Input: part model. Units: mm. Frame: model coordinates. Coordinates: 2 decimals unless noted, no trailing zeros. Loops run counter-clockwise (first coordinate to the right, second up) from the corner with the lowest first, then second, coordinate; pieces in that order, holes last.
(1) Section A-A, the plane y = 0. Return loops of the section in (x, z), then the cut area to 3 significant figures.
(2) Section C-C, the plane x = 162.5. Return loops of the section in (y, z), then the cut area to 3 significant figures.
(3) Contact query for flat-ended pins moving along their axis: P1, Ø2, axis at y = 5, z = -4, coming from the -X side; P2, Ø1.5, axis at x = 68, z = 4.5, coming from the -Y side; P3, Ø2, axis at x = 143, y = 6.5, coming from the -Z side; P4, Ø4, axis at x = 86, y = 3, coming from the -Z side. Output: stop coordinate, or through.
(4) Line query: L1, parallel to Z at x = 170.5, y = 0; L2, parallel to Z at x = 136.5, y = -4.5; L3, parallel to Y at x = 136.5, z = -6.5. Output: solid intervals per line, ascending.
Autodesk Inventor part; units mm, degrees
ref_plane "tube_front_XY" through (0, 0, 0) normal (1, 0, 0) x (0, 0, -1)
ref_plane "tube_front_YZ" through (0, 0, 0) normal (0, 0, -1) x (0, 1, 0)
ref_plane "tube_front_ZX" through (0, 0, 0) normal (0, 1, 0) x (1, 0, 0)
sketch "Sketch_1" plane through (0, 0, 0) normal (0, 0, 1) x (1, 0, 0)
  line L0 (260.4897, 0) -> (0, 0)
  arc A0 (-0.6395, 9.3472) -> (-0.6395, 9.1676) centre (-0.5497, 9.2574) ccw
  line L1 (-0.6395, 9.1676) -> (-0.381, 8.9091)
  line L2 (-0.381, 8.9091) -> (0, 8.9091)
  line L3 (0, 8.9091) -> (0.762, 9.671)
  line L4 (0.762, 9.671) -> (259.7277, 9.671)
  line L5 (259.7277, 9.671) -> (260.4897, 8.9091)
  line L6 (260.4897, 8.9091) -> (260.8707, 8.9091)
  line L7 (260.8707, 8.9091) -> (261.1292, 9.1676)
  arc A1 (261.1292, 9.1676) -> (261.1292, 9.3472) centre (261.0394, 9.2574) ccw
  line L8 (261.1292, 9.3472) -> (260.4443, 10.0321)
  arc A2 (260.4443, 10.0321) -> (259.9055, 10.2553) centre (259.9055, 9.4933) ccw
  line L9 (259.9055, 10.2553) -> (0.5842, 10.2553)
  arc A3 (0.5842, 10.2553) -> (0.0454, 10.0321) centre (0.5842, 9.4933) ccw
  line L10 (0.0454, 10.0321) -> (-0.6395, 9.3472)
revolve "Revolution1" add sketch "Sketch_1" angle 360 about axis through (260.4897, 0, 0) along (1, 0, 0)
ref_plane "tube_front_XY" through (0, 0, 0) normal (1, 0, 0) x (0, 0, -1)
ref_plane "tube_front_YZ" through (0, 0, 0) normal (0, 0, -1) x (0, 1, 0)
ref_plane "tube_front_ZX" through (0, 0, 0) normal (0, 1, 0) x (1, 0, 0)
ref_plane "tube_rear_XY" through (260.4897, 0, 0) normal (1, 0, 0) x (0, 0, -1)
ref_plane "tube_rear_YZ" through (260.4897, 0, 0) normal (0, 0, -1) x (0, 1, 0)
ref_plane "tube_rear_ZX" through (260.4897, 0, 0) normal (0, 1, 0) x (1, 0, 0)
ref_plane "cp1_XY" through (130.2449, 10.2553, 0) normal (1, 0, 0) x (0, 0, -1)
ref_plane "cp1_YZ" through (130.2449, 10.2553, 0) normal (0, 0, -1) x (0, 1, 0)
ref_plane "cp1_ZX" through (130.2449, 10.2553, 0) normal (0, 1, 0) x (1, 0, 0)
ref_plane "cp2_XY" through (130.2449, 0, -10.2553) normal (1, 0, 0) x (0, 0, -1)
ref_plane "cp2_YZ" through (130.2449, 0, -10.2553) normal (0, 0, -1) x (0, 1, 0)
ref_plane "cp2_ZX" through (130.2449, 0, -10.2553) normal (0, 1, 0) x (1, 0, 0)
ref_plane "cp3_XY" through (130.2449, -10.2553, 0) normal (1, 0, 0) x (0, 0, -1)
ref_plane "cp3_YZ" through (130.2449, -10.2553, 0) normal (0, 0, -1) x (0, 1, 0)
ref_plane "cp3_ZX" through (130.2449, -10.2553, 0) normal (0, 1, 0) x (1, 0, 0)
ref_plane "cp4_XY" through (130.2449, 0, 10.2553) normal (1, 0, 0) x (0, 0, -1)
ref_plane "cp4_YZ" through (130.2449, 0, 10.2553) normal (0, 0, -1) x (0, 1, 0)
ref_plane "cp4_ZX" through (130.2449, 0, 10.2553) normal (0, 1, 0) x (1, 0, 0)
properties part number "04R-10.25550" material "Stainless Steel"
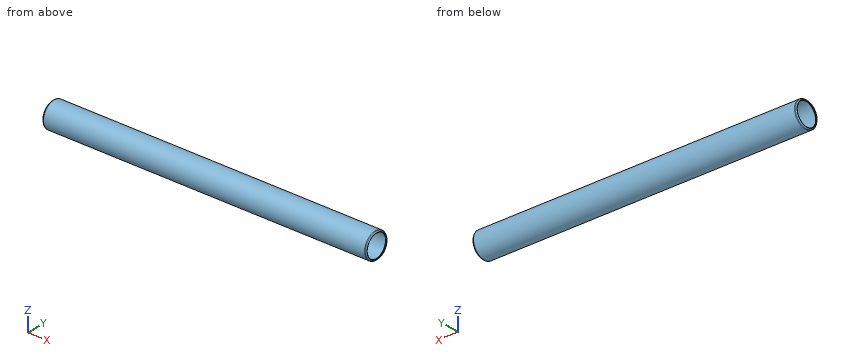
Report:
1. outline: (-0.64, -9.35) - (0.05, -10.03) arc R0.76 ccw to (0.58, -10.26) - (259.91, -10.26) arc R0.76 ccw to (260.44, -10.03) - (261.13, -9.35) arc R0.13 ccw to (261.13, -9.17) - (260.87, -8.91) - (260.49, -8.91) - (259.73, -9.67) - (0.76, -9.67) - (0, -8.91) - (-0.38, -8.91) - (-0.64, -9.17) arc R0.13 ccw to start; (-0.64, 9.17) - (-0.38, 8.91) - (0, 8.91) - (0.76, 9.67) - (259.73, 9.67) - (260.49, 8.91) - (260.87, 8.91) - (261.13, 9.17) arc R0.13 ccw to (261.13, 9.35) - (260.44, 10.03) arc R0.76 ccw to (259.91, 10.26) - (0.58, 10.26) arc R0.76 ccw to (0.05, 10.03) - (-0.64, 9.35) arc R0.13 ccw to start
1. area: 307 mm2
2. outline: circle Ø20.51 at (0, 0); hole circle Ø19.34 at (0, 0)
2. area: 36.6 mm2
3. P1: passes through
3. P2: stops at y = -9.55
3. P3: stops at z = -8.66
3. P4: stops at z = -10.21
4. L1: z = -10.26 to -9.67, 9.67 to 10.26
4. L2: z = -9.22 to -8.56, 8.56 to 9.22
4. L3: y = -7.93 to -7.16, 7.16 to 7.93
